Could you check a few things on this model? Use its own coordinates, in mm. A direction names the side the tool comes from. Round coordinates to 2 decimals unless told otherwise and drop trailing zeros. Loops run counter-clockwise (first coordinate to the right, second up) from the corner with the lowest first, then second, coordinate; pieces in that order, holes last.
Autodesk Fusion 360 part; units mm, degrees
sketch "Sketch1" plane through (0, 0, 0) normal (0, 0, 1) x (1, 0, 0) in component "funnel"
  circle A0 centre (0, 0) radius 17.75
  dimension "d1" = 35.5
extrude "Extrude2" add sketch "Sketch1" along normal blind 11 in component "funnel"
ref_plane "WorkPlane1" through (0, 0, -10) normal (0, 0, 1) x (1, 0, 0) in component "funnel"
sketch "Sketch2" plane through (0, 0, -10) normal (0, 0, 1) x (1, 0, 0) in component "funnel"
  circle A0 centre (0, 0) radius 8.75
  circle A1 centre (0, 0) radius 9.75
  circle A2 centre (0, 0) radius 17.75
  dimension "d7" = 1
  dimension "d10" = 9
loft "Loft1" add profiles "Sketch1", "Sketch2" section 1 section 2 contours A0 | A1 in component "funnel"
extrude "Extrude3" add 1 faces at (1.6592, 0.958, -10) along direction (0, 0, -1) blind 20 in component "funnel"
fillet "Fillet1" radius 5.5 2 edges at (-9.0902, -3.5258, -10) (-16.5488, -6.4187, 0) in component "funnel"
shell "Shell1" thickness 1 outward yes removed faces 2 at (2.6955, 3.38, 11) at (1.6592, 0.958, -30) in component "funnel"
component "funnel" placed x (1, 0, 0) y (0, 1, 0) z (0, 0, 1) at (0, 0, 0)
Item 1: For faces 1 (the cylindrical face through (-1.4, 10.66, -20.84)), 2 (the cylindrical face through (16.396, 6.798, 6.401)), 3 (the flat face through (2, -10, -30)), which set-ups out of +Z, -Z, +X, -X, +Y, -Y let a thin tool reach every point of the face, with its end or its side?
Results list:
face 1: -Z
face 2: +Z
face 3: -Z, +X, -X, +Y, -Y
Item 2: If we section it at A-A, the plane z = -24: Please give me the cut outline in (x, y), then the cut area to 3 significant figures.
Results list:
outline: circle Ø21.5 at (0, 0); hole circle Ø19.5 at (0, 0)
area: 64.4 mm2
Item 3: Will these pins go through, and if not, where does the flat tip stop? pin 1 (1.5 mm diameter, centred on y = 8.5, z = -24, fed in from +X); pin 2 (12 mm diameter, centred on x = -5.5, z = -15.5, fed in from -Y); pin 3 (1 mm diameter, centred on y = 7.5, z = -21.5, fed in from -X).
Results list:
pin 1: stops at x = 7.45
pin 2: stops at y = -10.77
pin 3: stops at x = -8.16
Item 4: If we section it at B-B, the plane z = -4.5: Please give me the cut outline in (x, y).
Results list:
outline: circle Ø30.86 at (0, 0); hole circle Ø28.3 at (0, 0)
Item 5: If I drill on line 1 along Y through (x, z) = (0, -17.75); line 2 along Y through (x, z) = (0, 4.5), over which ranges is the centre line in solid material (lowest first)?
Results list:
line 1: y = -10.75 to -9.75, 9.75 to 10.75
line 2: y = -18.75 to -17.75, 17.75 to 18.75
Item 6: We'd pull the mould along X, two halves only. Please class faces 4 (the cylindrical face through (9.3, 2.93, -20.84)), 5 (the cylindrical face through (17.884, -5.632, 6.401)), 6 (the flat face through (17, -7, 11)): released by +X, released by -X, zero draft, split by the parting line, or undercut.
Results list:
face 4: undercut
face 5: split by the parting line
face 6: zero draft
